```python
from build123d import *

# Parameters (mm, degrees)
SKETCH1_R           = 22.225
BOSS_EXTRUDE1_DEPTH = 38.1
SKETCH2_R           = 18.5039
CUT_EXTRUDE1_DEPTH  = 8.9916
CUT_EXTRUDE2_START  = -8.9916
SKETCH4_R           = 18.5039
CUT_EXTRUDE2_DEPTH  = 8.9916
SKETCH5_R           = 17.145
CUT_EXTRUDE3_DEPTH  = 43.839236694


with BuildPart() as part:
    # Sketch1 → Boss-Extrude1 (new body)
    with BuildSketch(Plane(origin=(0, 0, 0), x_dir=(1, 0, 0), z_dir=(0, 1, 0))):
        with Locations(Location((0, 0, 0), (0, 0, 90))):
            Circle(SKETCH1_R)
    extrude(amount=BOSS_EXTRUDE1_DEPTH)

    # Sketch2 → Cut-Extrude1 (cut)
    with BuildSketch(Plane(origin=(0, 38.1, 0), x_dir=(1, 0, 0), z_dir=(0, 1, 0))):
        with Locations(Location((0, 0, 0), (0, 0, 270))):
            Circle(SKETCH2_R)
    extrude(amount=-CUT_EXTRUDE1_DEPTH, mode=Mode.SUBTRACT)

    # Sketch4 → Cut-Extrude2 (cut)
    with BuildSketch(Plane.XZ.offset(CUT_EXTRUDE2_START)):
        with Locations(Location((0, 0, 0), (0, 0, 90))):
            Circle(SKETCH4_R)
    extrude(amount=CUT_EXTRUDE2_DEPTH, mode=Mode.SUBTRACT)

    # Sketch5 → Cut-Extrude3 (cut, through all)
    with BuildSketch(Plane.XZ.offset(-8.9916)):
        with Locations(Location((0, 0, 0), (0, 0, 270))):
            Circle(SKETCH5_R)
    extrude(amount=-CUT_EXTRUDE3_DEPTH, mode=Mode.SUBTRACT)


solid = part.part
```
Design review of the part built by this model. Coordinates are the model's own, in mm. A direction names the side the tool comes from. Give positions to 0.01 mm unless a question says otherwise; leave off trailing zeros. Order: outer loops, then holes, each group sorted by start corner. A loop starts at its lowest first (then second) coordinate and runs counter-clockwise, first axis right, second up. Notation, with made-up numbers: (-7.75, 89.5) -> (44.25, 89.5) arc R18 ccw to (44.25, 107.5) -> close; hole circle Ø8 at (30.25, 43.25). An arc over 180 degrees is marked (long way). Write each question's results on one line, items separated by ' | '. Start each with the question number.
Q1. Add section B-B on x = 0. Give the boundary of the cut face in (y, z) (3 decimals), and give its area (3 significant figures).
Q2. Mouldability with a two-part tool opening along X and no side actions: class faces 4 (the cylindrical face through (-18.74, 18.78, -11.95)), 5 (the cylindrical face through (5.15, 18.909, -16.353)), 6 (the flat face through (-17, 38.1, 8)) as +X half, -X half, draft (parallel to the pull), parting line (faces both ways), or undercut.
Q3. Wall thickness on L1, parallel to X at y = 5, z = 0 (3 decimals); L2, parallel to X at y = 22, z = 0 (3 decimals); L3, parallel to Z at x = 2, y = 26.5: over which ranges is each line inside the solid? List them lowest first. Write a range as from..to.
Q4. Add section A-A on z = 0. Give the boundary of the cut face in (x, y) (3 decimals), and give its area (3 significant figures).
Q5. Add section D-D on z = -19.5. Give the boundary of the cut face in (x, y).
Q6. Machinability: for faces 1 (the flat face through (-12.25, 29.108, 12.25)), 2 (the flat face through (-17, 0, 8)), 3 (the cylindrical face through (18.064, 4.559, -4.011)), which of the approach directions +Z, -Z, +X, -X, +Y, -Y give a long, thin tool a straight path to every point of the face, cutting with its end or side? Answer none if there is none.
Q7. Add section C-C on y = 12. Give the boundary of the cut face in (x, z) (3 decimals).
Q8. For pin 1 (3 mm diameter, centred on x = 6.5, y = 9.5, fed in from +Z); pin 2 (12 mm diameter, centred on y = 33.5, z = -14, fed in from -X); pin 3 (1 mm diameter, centred on y = 14, z = 13, fed in from +X); pin 4 (10 mm diameter, centred on x = -5, z = -5.5, fed in from +Y), all flat-tipped, find the tip position at first contact; note any pin that passes through.
Found:
1) outline: (0, -22.225) -> (38.1, -22.225) -> (38.1, -18.504) -> (29.108, -18.504) -> (29.108, -17.145) -> (8.992, -17.145) -> (8.992, -18.504) -> (0, -18.504) -> close; (0, 18.504) -> (8.992, 18.504) -> (8.992, 17.145) -> (29.108, 17.145) -> (29.108, 18.504) -> (38.1, 18.504) -> (38.1, 22.225) -> (0, 22.225) -> close | area: 338 mm2
2) face 4: parting line | face 5: undercut | face 6: draft
3) L1: x = -22.225..-18.504, 18.504..22.225 | L2: x = -22.225..-17.145, 17.145..22.225 | L3: z = -22.13..-17.03, 17.03..22.13
4) outline: (-22.225, 0) -> (-18.504, 0) -> (-18.504, 8.992) -> (-17.145, 8.992) -> (-17.145, 29.108) -> (-18.504, 29.108) -> (-18.504, 38.1) -> (-22.225, 38.1) -> close; (17.145, 8.992) -> (18.504, 8.992) -> (18.504, 0) -> (22.225, 0) -> (22.225, 38.1) -> (18.504, 38.1) -> (18.504, 29.108) -> (17.145, 29.108) -> close | area: 338 mm2
5) outline: (-10.66, 0) -> (10.66, 0) -> (10.66, 38.1) -> (-10.66, 38.1) -> close
6) face 1: +Y | face 2: +Z, -Z, +X, -X, -Y | face 3: -Y
7) outline: circle Ø44.45 at (0, 0); hole circle Ø34.29 at (0, 0)
8) pin 1: stops at z = 21.66 | pin 2: stops at x = -20.74 | pin 3: stops at x = 18.38 | pin 4: passes through
